The listing builds one solid part. Answer for the finished solid, in the listing's coordinates (mm). Face numbers are marked on the shaded views. A direction names the side the tool comes from. Round coordinates to 2 decimals unless told otherwise and drop trailing zeros. Order: outer loops, then holes, each group sorted by start corner. A loop starts at its lowest first (then second) coordinate and runs counter-clockwise, first axis right, second up. Notation, with made-up numbers: (75.5, 6.5) - (132.5, 6.5) arc R25 ccw to (132.5, 22.5) - close; hole circle Ø2 at (58, 11). An arc over 180 degrees is marked (long way). One line per item, written item: value. Start each with the question number.
1. Section D-D, the plane x = 401.5 is taken. Give the vertices of the cut face in (y, z).
2. A tool of negligible diameter and unlimited length cuts with its end or side. For the marked faces 1, 2 and 3, from which of +Z, -Z, +X, -X, +Y, -Y can it reach the whole face along a straight path? Write none if from no direction.
3. For a pull along Y with two mould halves and no side action, classify the marked faces 4, 5 and 6 as released by +Y, released by -Y, zero draft, split by the parting line, or undercut.
4. Section B-B, the plane y = 642.85 is taken. Give the vertices of the cut face in (x, z), then the cut area to 3 significant figures.
5. Flat-ended cylindrical pins translate along their axes: P1, Ø5, axis at x = 398.75, y = 642.85, coming from the -Z side; P2, Ø3, axis at x = 395.5, y = 653.5, coming from the +Z side; P3, Ø2.5, axis at x = 398.75, y = 662.85, coming from the +Z side; P4, Ø1.1, axis at y = 652, z = 48.5, coming from the +X side. Find the tip coordinate at first contact, or state that the pin passes through.
6. Section C-C, the plane z = 50.2 is taken. Give the vertices of the cut face in (x, y).
7. Section A-A, the plane x = 398.75 is taken. Give the vertices of the cut face in (y, z).
8. Straight lines are drawn through the part: line 1 (Y direction, x = 398.75, z = 52.3); line 2 (X direction, y = 662.85, z = 50.45); line 3 (Y direction, x = 400.75, z = 51.5). For each, find the intervals that lie inside material, in ascending order.
from build123d import *

# Parameters (mm, degrees)
CYLINDER073_R          = 2.2
CYLINDER073_DEPTH      = 20
CYLINDER074_R          = 2.2
CYLINDER074_DEPTH      = 20
CYLINDER072_R          = 4
CYLINDER072_DEPTH      = 6.5
CYLINDER071_W          = 6
CYLINDER071_H          = 11
CYLINDER071_ANGLE      = 180
BOX054_W               = 30
BOX054_H               = 3.7
BOX054_DEPTH           = 13
CUT090_ROLL_ANGLE      = 90
CUT090_PLACEMENT_ANGLE = -90


with BuildPart() as zylinder062:
    # Cylinder073 → Cylinder073 (new body)
    with BuildSketch(Plane(origin=(-10, 9, 5), x_dir=(1, 0, 0), z_dir=(0, -1, 0))):
        Circle(CYLINDER073_R)
    extrude(amount=CYLINDER073_DEPTH)


with BuildPart() as zylinder063:
    # Cylinder074 → Cylinder074 (new body)
    with BuildSketch(Plane(origin=(10, 9, 5), x_dir=(1, 0, 0), z_dir=(0, -1, 0))):
        Circle(CYLINDER074_R)
    extrude(amount=CYLINDER074_DEPTH)


with BuildPart() as zylinder061:
    # Cylinder072 → Cylinder072 (new body)
    with BuildSketch(Plane.XY.offset(5.8)):
        Circle(CYLINDER072_R)
    extrude(amount=CYLINDER072_DEPTH)


with BuildPart() as zylinder060:
    # Cylinder071 → Cylinder071 (revolve)
    with BuildSketch(Plane(origin=(0, 0, 0), x_dir=(-1, 0, 0), z_dir=(0, 1, 0))):
        with Locations((3, 5.5)):
            Rectangle(CYLINDER071_W, CYLINDER071_H)
    revolve(axis=Axis((0, 0, 0), (0, 0, 1)), revolution_arc=CYLINDER071_ANGLE)


with BuildPart() as y_drive_mount_top004:
    # Box054 → Box054 (new body)
    with BuildSketch(Plane(origin=(-15, -3.7, -2), x_dir=(1, 0, 0), z_dir=(0, 0, 1))):
        with Locations((15, 1.85)):
            Rectangle(BOX054_W, BOX054_H)
    extrude(amount=BOX054_DEPTH)

    # Fusion041: union Zylinder060
    add(zylinder060.part)

    # Cut081: cut Zylinder061
    add(zylinder061.part, mode=Mode.SUBTRACT)

    # Cut082: cut Zylinder063
    add(zylinder063.part, mode=Mode.SUBTRACT)

    # Cut090: cut Zylinder062
    add(zylinder062.part, mode=Mode.SUBTRACT)


with BuildPart() as y_drive_mount_top004_1:
    # Cut090 roll: moved
    add(y_drive_mount_top004.part.rotate(Axis((0, 0, 0), (1, 0, 0)), CUT090_ROLL_ANGLE))


with BuildPart() as y_drive_mount_top004_2:
    # Cut090 placement: moved
    add(y_drive_mount_top004_1.part.moved(Location((403.75, 652.85, 53.2))).rotate(Axis((403.75, 652.85, 53.2), (0, 0, 1)), CUT090_PLACEMENT_ANGLE))


solid = y_drive_mount_top004_2.part
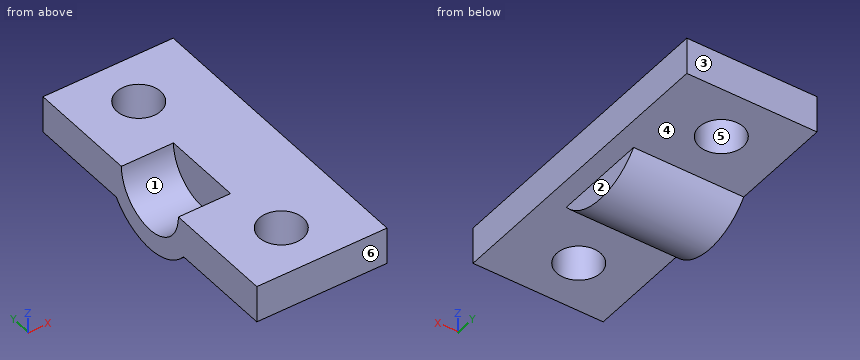
Answer list:
1. outline: (637.85, 49.5) - (648.13, 49.5) arc R6 ccw to (657.57, 49.5) - (667.85, 49.5) - (667.85, 53.2) - (637.85, 53.2) - close
2. face 1: +Z, -X
2. face 2: -Z, +X, +Y, -Y
2. face 3: +Z, -Z, +X, -X, +Y
3. face 4: zero draft
3. face 5: undercut
3. face 6: released by -Y
4. outline: (392.75, 49.5) - (396.55, 49.5) - (396.55, 53.2) - (392.75, 53.2) - close; (400.95, 49.5) - (405.75, 49.5) - (405.75, 53.2) - (400.95, 53.2) - close
4. area: 31.8 mm²
5. P1: stops at z = 49.5
5. P2: stops at z = 49.83
5. P3: passes through
5. P4: stops at x = 403.75
6. outline: (392.75, 637.85) - (405.75, 637.85) - (405.75, 667.85) - (392.75, 667.85) - (392.75, 655.5) - (397.95, 655.5) - (397.95, 650.2) - (392.75, 650.2) - close; hole circle Ø4.4 at (398.75, 642.85); hole circle Ø4.4 at (398.75, 662.85)
7. outline: (637.85, 49.5) - (640.65, 49.5) - (640.65, 53.2) - (637.85, 53.2) - close; (645.05, 49.5) - (648.13, 49.5) arc R6 ccw to (657.57, 49.5) - (660.65, 49.5) - (660.65, 53.2) - (645.05, 53.2) - close; (665.05, 49.5) - (667.85, 49.5) - (667.85, 53.2) - (665.05, 53.2) - close
8. line 1: y = 637.85 to 640.65, 645.05 to 660.65, 665.05 to 667.85
8. line 2: x = 392.75 to 396.55, 400.95 to 405.75
8. line 3: y = 637.85 to 641.93, 643.77 to 661.93, 663.77 to 667.85
